Autodesk Inventor part; units mm, degrees
ref_plane "YZ Plane" through (0, 0, 0) normal (1, 0, 0) x (0, 1, 0)
ref_plane "XZ Plane" through (0, 0, 0) normal (0, 1, 0) x (-1, 0, 0)
ref_plane "XY Plane" through (0, 0, 0) normal (0, 0, 1) x (1, 0, 0)
sketch "Esquisse1" plane through (0, 0, 0) normal (0, 1, 0) x (-1, 0, 0)
  circle A0 centre (0, 0) radius 15
  dimension "d0" = 30
extrude "Extrusion1" add sketch "Esquisse1" along normal blind 17
chamfer "Chanfrein1" distance 1 angle 86 1 edges at (15, 17, 0) measured on face at (-3.8878, 17, -2.119)
fillet "Congé1" radius 1.5 1 edges at (14, 17, 0)
sketch "Esquisse2" plane through (0, 17, 0) normal (0, 1, 0) x (1, 0, 0)
  circle A0 centre (0, 0) radius 8
  dimension "d7" = 16
extrude "Extrusion2" cut sketch "Esquisse2" against normal blind 9
fillet "Congé2" radius 1.5 1 edges at (-8, 17, 0)
sketch "Esquisse3" plane through (0, 0, 0) normal (0, -1, 0) x (1, 0, 0)
  circle A0 centre (0, 0) radius 2
  dimension "d11" = 4
extrude "Extrusion3" cut sketch "Esquisse3" against normal blind 9
mirror "Symétrie1" about plane through (0, 0, 0) normal (0, -1, 0) of "Extrusion1", "Chanfrein1", "Congé1", "Extrusion2", "Congé2", "Extrusion3"
properties part number "Pied" material "Caoutchouc"
Here's how the part is built. I have some questions about the finished solid (model axes, mm). A direction names the side the tool comes from. Round coordinates to 2 decimals unless told otherwise and drop trailing zeros. Order: outer loops, then holes, each group sorted by start corner. A loop starts at its lowest first (then second) coordinate and runs counter-clockwise, first axis right, second up. Notation, with made-up numbers: M 7,64.25 L 50,64.25 A23 cw 50,91.25 Z; hole C 48.25,52.25 d11. An arc over 180 degrees is marked long. Use CSV: the item, a comma, the result in double quotes.
1) I want a section at C-C (y = 7). List the corners of the cut face in (x, z) for me, then the cut area to 3 significant figures.
Taken from the geometry:
outline,"C 0,0 d29.4; hole C 0,0 d4"
area,"666 mm^2"
2) I want a section at D-D (y = 2). List the corners of the cut face in (x, z) for me.
Taken from the geometry:
outline,"C 0,0 d30; hole C 0,0 d4"
3) On a 3-axis mill with a long thin cutter (end or side, diameter ignored), from which of +Z, -Z, +X, -X, +Y, -Y can I reach the whole of each face in a straight line? I mean faces 1 (the flat face through (2, 8, 2)), 2 (the cylindrical face through (0, 0, -2)), 3 (the cylindrical face through (-1.73, -11.8, -7.81)). Say none if no direction works.
Taken from the geometry:
face 1,"+Y"
face 2,"+Y, -Y"
face 3,"-Y"
4) I need wall thicknesses on line 1 along Z through (x, y) = (0, -0.75); line 2 along X through (y, z) = (-12.75, 0); line 3 along X through (y, z) = (11, -7). Which ranges of each line are inside material? Lowest first, please. Write a range as [from, to].
Taken from the geometry:
line 1,"[-15, -2], [2, 15]"
line 2,"[-14.3, -8], [8, 14.3]"
line 3,"[-12.61, -3.87], [3.87, 12.61]"
5) I'm going to push flat-ended pins straight in: P1, Ø12, axis at x = 11, y = 11.5, coming from the +Z side; P2, Ø4, axis at x = -4, y = 12.5, coming from the +Z side; P3, Ø1, axis at x = 11.5, y = -6.5, coming from the -Z side. Where does each tip first touch, or does it pass through?
Taken from the geometry:
P1,"z = 13.53"
P2,"z = 14.21"
P3,"z = -9.81"
6) I want a section at A-A (z = 0). List the corners of the cut face in (x, y) for me, then the cut area to 3 significant figures.
Taken from the geometry:
outline,"M -15,-2.7 L -14.1,-15.6 A1.5 ccw -12.6,-17 L -9.5,-17 A1.5 ccw -8,-15.5 L -8,-8 L -2,-8 L -2,8 L -8,8 L -8,15.5 A1.5 ccw -9.5,17 L -12.6,17 A1.5 ccw -14.1,15.6 L -15,2.7 Z; M 2,-8 L 8,-8 L 8,-15.5 A1.5 ccw 9.5,-17 L 12.6,-17 A1.5 ccw 14.1,-15.6 L 15,-2.7 L 15,2.7 L 14.1,15.6 A1.5 ccw 12.6,17 L 9.5,17 A1.5 ccw 8,15.5 L 8,8 L 2,8 Z"
area,"636 mm^2"
7) If we mould it in two halves opening along X, with no side actions, what happens to faces 4 (the cylindrical face through (-1.73, 11.8, 7.81)), 5 (the cylindrical face through (14.985, 0.038, 0.66)), 6 (the flat face through (-2, -8, 2)), 7 (the flat face through (4.7, 17, 8.5))? For each: pulls with the +X half, pulls with the -X half, needs draft (parallel to the pull), parting line crosses it, or undercut.
Taken from the geometry:
face 4,"undercut"
face 5,"parting line crosses it"
face 6,"undercut"
face 7,"needs draft"
8) I want a section at B-B (x = 0). List the corners of the cut face in (y, z) for me.
Taken from the geometry:
outline,"M -17,-12.6 A1.5 ccw -15.6,-14.1 L -2.7,-15 L 2.7,-15 L 15.6,-14.1 A1.5 ccw 17,-12.6 L 17,-9.5 A1.5 ccw 15.5,-8 L 8,-8 L 8,-2 L -8,-2 L -8,-8 L -15.5,-8 A1.5 ccw -17,-9.5 Z; M -17,9.5 A1.5 ccw -15.5,8 L -8,8 L -8,2 L 8,2 L 8,8 L 15.5,8 A1.5 ccw 17,9.5 L 17,12.6 A1.5 ccw 15.6,14.1 L 2.7,15 L -2.7,15 L -15.6,14.1 A1.5 ccw -17,12.6 Z"
